```python
from build123d import *

# Parameters (mm, degrees)
F0_R     = 2.085
F0_R_2   = 2.15
F0_W     = 3.175
F0_H     = 23
F1_DEPTH = 3.175


with BuildPart() as f1:
    # F0 (on Top) → F1 (new body)
    with BuildSketch(Plane.XY):
        with BuildLine():
            Line((-38, -41.9637251374), (0, -41.9637251374))
            Line((0, -41.9637251374), (38, -41.9637251374))
            Line((38, -41.9637251374), (37.9384113545, 1.9986380357))
            Line((37.9384113545, 1.9986380357), (52.9251351953, 1.9986380357))
            Line((52.9251351953, 1.9986380357), (52.9251351953, 31.9986380357))
            Line((52.9251351953, 31.9986380357), (37.9251351953, 31.9986380357))
            Line((37.9251351953, 31.9986380357), (49.9251351953, 76.4752441225))
            Line((49.9251351953, 76.4752441225), (47.2431264601, 76.4752441225))
            ThreePointArc((47.2431264601, 76.4752441225), (39.0233041791, 77.3289221795), (31.1543359938, 79.8535180391))
            ThreePointArc((31.1543359938, 79.8535180391), (0, 86.3952080993), (-31.1543359938, 79.8535180391))
            ThreePointArc((-31.1543359938, 79.8535180391), (-39.0233041791, 77.3289221795), (-47.2431264601, 76.4752441225))
            Line((-47.2431264601, 76.4752441225), (-49.9251351953, 76.4752441225))
            Line((-49.9251351953, 76.4752441225), (-37.9251351953, 31.9986380357))
            Line((-37.9251351953, 31.9986380357), (-52.9251351953, 31.9986380357))
            Line((-52.9251351953, 31.9986380357), (-52.9251351953, 1.9986380357))
            Line((-52.9251351953, 1.9986380357), (-37.9384113545, 1.9986380357))
            Line((-37.9384113545, 1.9986380357), (-38, -41.9637251374))
        make_face()
        with Locations((-32.1168240318, -36.3078415394)):
            Circle(F0_R, mode=Mode.SUBTRACT)
        with Locations((-32.1168240318, -21.7403415394)):
            Circle(F0_R, mode=Mode.SUBTRACT)
        with Locations((-47.1168240318, 5.6010650516)):
            Circle(F0_R, mode=Mode.SUBTRACT)
        with Locations((-32.1168240318, -7.1728415394)):
            Circle(F0_R, mode=Mode.SUBTRACT)
        with Locations((-32.1168240318, 5.6010650516)):
            Circle(F0_R, mode=Mode.SUBTRACT)
        with Locations((32.1168240318, -36.3078415394)):
            Circle(F0_R, mode=Mode.SUBTRACT)
        with Locations((32.1168240318, -21.7403415394)):
            Circle(F0_R, mode=Mode.SUBTRACT)
        with Locations((32.1168240318, -7.1728415394)):
            Circle(F0_R, mode=Mode.SUBTRACT)
        with Locations((32.1168240318, 5.6010650516)):
            Circle(F0_R, mode=Mode.SUBTRACT)
        with BuildLine():
            ThreePointArc((49.2018240318, 5.6010650516), (45.6425063931, 4.1267474129), (47.1168240318, 7.6860650516))
            ThreePointArc((47.1168240318, 7.6860650516), (48.5911416706, 7.0753826904), (49.2018240318, 5.6010650516))
        make_face(mode=Mode.SUBTRACT)
        with Locations((-47.1168240318, 27.9740650516)):
            Circle(F0_R, mode=Mode.SUBTRACT)
        with Locations((-32.1168240318, 27.9742324866)):
            Circle(F0_R, mode=Mode.SUBTRACT)
        with Locations((-16.75, 47.0501706004)):
            Circle(F0_R_2, mode=Mode.SUBTRACT)
        with Locations((-36.0875, 60.3372221589)):
            Rectangle(F0_W, F0_H, mode=Mode.SUBTRACT)
        with Locations((-16.75, 80.0501706004)):
            Circle(F0_R_2, mode=Mode.SUBTRACT)
        with Locations((16.75, 47.0501706004)):
            Circle(F0_R_2, mode=Mode.SUBTRACT)
        with Locations((32.1168240318, 27.9742324866)):
            Circle(F0_R, mode=Mode.SUBTRACT)
        with BuildLine():
            ThreePointArc((47.1168240318, 25.8890650516), (45.6425063931, 29.4483826904), (49.2018240318, 27.9740650516))
            ThreePointArc((49.2018240318, 27.9740650516), (48.5911416706, 26.4997474129), (47.1168240318, 25.8890650516))
        make_face(mode=Mode.SUBTRACT)
        with Locations((16.75, 80.0501706004)):
            Circle(F0_R_2, mode=Mode.SUBTRACT)
        with Locations((36.0875, 60.3372221589)):
            Rectangle(F0_W, F0_H, mode=Mode.SUBTRACT)
    extrude(amount=F1_DEPTH)


solid = f1.part
```
Design review of the part built by this model. Coordinates are the model's own, in mm. A direction names the side the tool comes from. Give positions to 0.01 mm unless a question says otherwise; leave off trailing zeros. Order: outer loops, then holes, each group sorted by start corner. A loop starts at its lowest first (then second) coordinate and runs counter-clockwise, first axis right, second up. Notation, with made-up numbers: (10, 9.25) -> (53, 9.25) arc R23 cw to (53, 33.25) -> close; hole circle Ø8 at (6, 65). An arc over 180 degrees is marked (long way). Write each question's results on one line, items separated by ' | '. Start each with the question number.
Q1. Add section B-B on x = -16.75. Give the boundary of the cut face in (y, z) (3 decimals), and give its area (3 significant figures).
Q2. Mouldability with a two-part tool opening along X and no side actions: class faces 1 (the cylindrical face through (39.137, 77.305, 1.565)), 2 (the flat face through (37.675, 60, 2)), 3 (the cylindrical face through (17.74, 78.14, 1.57)), 4 (the flat face through (49, 76.475, 2)) as +X half, -X half, draft (parallel to the pull), parting line (faces both ways), or undercut.
Q3. Wall thickness on L1, parallel to X at y = 27.5, z = 2.15; L2, parallel to X at y = 68.5, z = 2.65 (3 decimals); L3, parallel to Y at x = -16.75, z = 2.4: over which ranges is each line inside the solid? List them lowest first. Write a range as from..to.
Q4. Add section A-A on y = 62. Give the boundary of the cut face in (x, z) (3 decimals), and give its area (3 significant figures).
Q5. Add section D-D on y = -11.5. Give the boundary of the cut face in (x, z) (3 decimals).
Q6. Add section C-C on z = 1.3. State how many separate pieces and enclosed holes the cut face has, and give its area (3 significant figures).
Q7. For pin 1 (3.5 mm diameter, centred on x = 32.12, y = -7.17, fed in from +Z); pin 2 (1 mm diameter, centred on y = 59, z = 1.5, fed in from -X); pin 3 (1 mm diameter, centred on y = -7, z = 1.5, fed in from -X); pin 4 (1.6 mm diameter, centred on x = 36, z = 2, fed in from +Y), all flat-tipped, find the tip position at first contact; note any pin that passes through.
Q8. Machinability: for faces 5 (the flat face through (-37.675, 60, 2)), 6 (the flat face through (46, 31.999, 2)), 7 (the flat face through (45, 1.999, 2)), 8 (the flat face through (-1, 23, 0)), which of the approach directions +Z, -Z, +X, -X, +Y, -Y give a long, thin tool a straight path to every point of the face, cutting with its end or side? Answer none if there is none.
Found:
1) outline: (-41.964, 0) -> (44.9, 0) -> (44.9, 3.175) -> (-41.964, 3.175) -> close; (49.2, 0) -> (77.9, 0) -> (77.9, 3.175) -> (49.2, 3.175) -> close; (82.2, 0) -> (84.562, 0) -> (84.562, 3.175) -> (82.2, 3.175) -> close | area: 374 mm2
2) face 1: +X half | face 2: undercut | face 3: undercut | face 4: draft
3) L1: x = -52.93..-49.15, -45.09..-34.15, -30.09..30.09, 34.15..45.09, 49.15..52.93 | L2: x = -47.773..-37.675, -34.5..34.5, 37.675..47.773 | L3: y = -41.96..44.9, 49.2..77.9, 82.2..84.56
4) outline: (-46.02, 0) -> (-37.675, 0) -> (-37.675, 3.175) -> (-46.02, 3.175) -> close; (-34.5, 0) -> (34.5, 0) -> (34.5, 3.175) -> (-34.5, 3.175) -> close; (37.675, 0) -> (46.02, 0) -> (46.02, 3.175) -> (37.675, 3.175) -> close | area: 272 mm2
5) outline: (-37.957, 0) -> (37.957, 0) -> (37.957, 3.175) -> (-37.957, 3.175) -> close
6) separate pieces: 1 | enclosed holes: 20 | area: 10,500 mm2
7) pin 1: passes through | pin 2: stops at x = -45.35 | pin 3: stops at x = -37.95 | pin 4: stops at y = 78.33
8) face 5: +Z, -Z | face 6: +Z, -Z, +X | face 7: +Z, -Z, +X, -Y | face 8: -Z, +X, -X, +Y, -Y
